Part model, mm, in its own coordinate system. A direction names the side the tool comes from. Coordinates: 2 decimals unless noted, no trailing zeros. Loops run counter-clockwise (first coordinate to the right, second up) from the corner with the lowest first, then second, coordinate; pieces in that order, holes last. Notation, with made-up numbers: (21.25, 35.5) - (72.25, 35.5) arc R17 ccw to (72.25, 39.5) - close; hole circle Ø7 at (27, 57). An arc over 180 degrees is marked (long way). Answer as CSV lines item,"result".
from build123d import *

# Parameters (mm, degrees)
SKETCH_1_W                = 100
SKETCH_1_H                = 60
EXTRUDE_1_DEPTH           = 6
SKETCH_2_R                = 11.5
SKETCH_2_R_2              = 1.5
CUT_EXTRUDE_1_DEPTH       = 10
SKETCH_3_R                = 18.5
CUT_EXTRUDE_2_DEPTH       = 4
HOLE_WIZARD_2_D           = 3.4
HOLE_WIZARD_2_CSINK_D     = 6.6
HOLE_WIZARD_2_CSINK_ANGLE = 90
CHAMFER_1_SIZE            = 10
HOLE_WIZARD_M3_1_D        = 2.5
HOLE_WIZARD_M3_1_DEPTH    = 7.5
HOLE_WIZARD_M3_1_TIP      = 0.751075774
SKETCH_16_R               = 1
CUT_EXTRUDE_3_DEPTH       = 6


with BuildPart() as part:
    # 草图1 → 凸台-拉伸1 (new body)
    with BuildSketch(Plane.XY):
        Rectangle(SKETCH_1_W, SKETCH_1_H)
    extrude(amount=EXTRUDE_1_DEPTH)

    # 草图2 → 切除-拉伸1 (cut)
    with BuildSketch(Plane.XY.offset(6)):
        with Locations((30, -8.8724e-05)):
            Circle(SKETCH_2_R)
        with Locations((40.606601718, 10.606512994)):
            Circle(SKETCH_2_R_2)
        with Locations((40.606601718, -10.606690441)):
            Circle(SKETCH_2_R_2)
        with Locations((19.393398282, 10.606512994)):
            Circle(SKETCH_2_R_2)
        with Locations((19.393398282, -10.606690441)):
            Circle(SKETCH_2_R_2)
    extrude(amount=-CUT_EXTRUDE_1_DEPTH, mode=Mode.SUBTRACT)

    # 草图3 → 切除-拉伸2 (cut)
    with BuildSketch(Plane.XY.offset(6)):
        with Locations((30, -8.8724e-05)):
            Circle(SKETCH_3_R)
    extrude(amount=-CUT_EXTRUDE_2_DEPTH, mode=Mode.SUBTRACT)

    # 打孔尺寸(%根据十字)槽半沉头木螺钉的类型2 (through all)
    with Locations(Plane(origin=(0, 0, 0), x_dir=(-1, 0, 0), z_dir=(0, 0, -1))):
        with Locations((47, -20), (47, 0), (47, 20)):
            CounterSinkHole(HOLE_WIZARD_2_D / 2, HOLE_WIZARD_2_CSINK_D / 2, counter_sink_angle=HOLE_WIZARD_2_CSINK_ANGLE)

    # 倒角1
    chamfer_1_edges = [part.edges().sort_by_distance(p)[0] for p in [
        (50, 30, 3),
        (50, -30, 3),
    ]]
    chamfer(chamfer_1_edges, length=CHAMFER_1_SIZE)

    # M3 螺纹孔1
    with Locations(Plane.XY.offset(6)):
        with Locations((-36, 5), (-26, -5)):
            Hole(HOLE_WIZARD_M3_1_D / 2, depth=HOLE_WIZARD_M3_1_DEPTH)
            with Locations((0, 0, -(HOLE_WIZARD_M3_1_DEPTH + HOLE_WIZARD_M3_1_TIP / 2))):  # 118° drill point
                Cone(0, HOLE_WIZARD_M3_1_D / 2, HOLE_WIZARD_M3_1_TIP, mode=Mode.SUBTRACT)

    # 草图16 → 切除-拉伸3 (cut)
    with BuildSketch(Plane.XY.offset(6)):
        with Locations((-2, 27)):
            Circle(SKETCH_16_R)
        with Locations((-11.5, 27)):
            Circle(SKETCH_16_R)
        with Locations((-11.5, -27)):
            Circle(SKETCH_16_R)
        with Locations((-2, -27)):
            Circle(SKETCH_16_R)
    extrude(amount=-CUT_EXTRUDE_3_DEPTH, mode=Mode.SUBTRACT)


solid = part.part
Q1. Saw through at C-C (y = 5). Give the cut face in (x, z), then the cut area to 3 significant figures.
Results:
outline,"(-50, 0) - (-37.25, 0) - (-37.25, 6) - (-50, 6) - close; (-34.75, 0) - (19.64, 0) - (19.64, 2) - (12.19, 2) - (12.19, 6) - (-34.75, 6) - close; (40.36, 0) - (50, 0) - (50, 6) - (47.81, 6) - (47.81, 2) - (40.36, 2) - close"
area,"401 mm^2"
Q2. Wall check: L1, parallel to Y at x = -47, z = 4.35; L2, parallel to Y at x = -11.5, z = 2.75; L3, parallel to X at y = -7, z = 1.55. Give the ranges that are in metal, low to high.
Results:
L1,"y = -30 to -21.7, -18.3 to -1.7, 1.7 to 18.3, 21.7 to 30"
L2,"y = -30 to -28, -26 to 26, 28 to 30"
L3,"x = -50 to 20.88, 39.12 to 50"
Q3. Saw through at D-D (z = 3.35). Count the separate pieces of the cut face and the enclosed holes in it, then the cut area to 3 significant figures.
Results:
separate pieces,"1"
enclosed holes,"10"
area,"4,780 mm^2"
Q4. Two-plate mould, pull along X, no slides. Class faces 1 (the face through (21.5, -8, 2)), 2 (the face through (-12, 0, 6)), 3 (the face through (45, -25, 3)): released by +X, released by -X, zero draft, split by the parting line, or undercut.
Results:
face 1,"undercut"
face 2,"zero draft"
face 3,"released by +X"
Q5. Which spindle directions (+Z, -Z, +X, -X, +Y, -Y) get a long thin tool onto all of the face, cutting with end or side? Do faces 4 (the face through (-1, 0, 0)), 5 (the face through (11.518, 0.813, 4.028)). Say none if no direction does.
Results:
face 4,"-Z, +X, -X, +Y, -Y"
face 5,"+Z"
Q6. Flat gauge pins, fed straight in: pin 1 (2.5 mm diameter, centred on x = 40.61, y = 10.61, fed in from +Z); pin 2 (4 mm diameter, centred on x = -47, y = -20, fed in from -Z); pin 3 (2 mm diameter, centred on y = 22, z = 2.5, fed in from +X); pin 4 (18.5 mm diameter, centred on x = 26, y = 5.5, fed in from +Z). Where does each tip first touch, or does it go through?
Results:
pin 1,"passes through"
pin 2,"stops at z = 1.3"
pin 3,"stops at x = 49"
pin 4,"stops at z = 2"
Q7. Saw through at A-A (x = -26). Give the cut face in (y, z), then the cut area to 3 significant figures.
Results:
outline,"(-30, 0) - (-6.25, 0) - (-6.25, 6) - (-30, 6) - close; (-3.75, 0) - (30, 0) - (30, 6) - (-3.75, 6) - close"
area,"345 mm^2"
Q8. Saw through at B-B (x = -2). Give the cut face in (y, z).
Results:
outline,"(-30, 0) - (-28, 0) - (-28, 6) - (-30, 6) - close; (-26, 0) - (26, 0) - (26, 6) - (-26, 6) - close; (28, 0) - (30, 0) - (30, 6) - (28, 6) - close"
